Can you work these out from the model? Positions are in its coordinate system, mm. Face numbers are marked on the shaded views. Give positions to 0.01 mm unless a question says otherwise; leave off trailing zeros. Loops run counter-clockwise (first coordinate to the right, second up) from the corner with the lowest first, then second, coordinate; pieces in that order, holes last. Notation, with made-up numbers: (16, 54) - (51, 54) arc R14 ccw to (51, 75) - close; hole circle Ø4 at (14, 65). An arc over 180 degrees is marked (long way). Answer as a JSON object with one key per item and string values. Group by question number.
Item 1: Thinking about a two-plate mould opening in Y: for the marked faces 1, 2 and 3, which applies, pulls with the +Y half, pulls with the -Y half, needs draft (parallel to the pull), parting line crosses it, or undercut?
Item 2: Suppose I cut it at C-C on x = 0. Write out the boundary of the cut face in (y, z).
Item 3: Suppose I cut it at D-D on x = 22. Write out the boundary of the cut face in (y, z), and give its area (3 significant figures).
Item 4: Will these pins go through, and if not, where does the flat tip stop? pin 1 (10 mm diameter, centred on x = 18.5, y = 19, fed in from -Z); pin 2 (4 mm diameter, centred on x = 15, y = 9, fed in from -Z); pin 3 (5 mm diameter, centred on y = 12.5, z = -2, fed in from -X).
Item 5: Suppose I cut it at B-B on y = 5.5. Count the separate pieces of the cut face and the enclosed holes in it, and give its area (3 significant figures).
Item 6: Please list where these lines run through material, in increasing order: L1, parallel to Z at x = 0, y = 14.5; L2, parallel to Y at x = 10.5, z = -23; L3, parallel to X at y = 21.5, z = -18.
Item 7: Suppose I cut it at A-A on z = 0. Write out the boundary of the cut face in (x, y).
from build123d import *

# Parameters (mm, degrees)
F0_R     = 25.4
F1_DEPTH = 6.35
F3_R     = 22.225
F4_DEPTH = 19.05
F5_R     = 25.4
F6_DEPTH = 6.35
F8_D     = 3.175
F9_D     = 12.7


with BuildPart() as f1:
    # F0 (on Front) → F1 (new body)
    with BuildSketch(Plane.XZ):
        with Locations((0.658478, 0)):
            Circle(F0_R)
    extrude(amount=F1_DEPTH)

    # F3 (on face) → F4 (join)
    with BuildSketch(Plane(origin=(0, 0, 0), x_dir=(-1, 0, 0), z_dir=(0, 1, 0))):
        with Locations((-0.658478, 0)):
            Circle(F3_R)
    extrude(amount=F4_DEPTH)

    # F5 (on face) → F6 (join)
    with BuildSketch(Plane(origin=(0, 19.05, 0), x_dir=(-1, 0, 0), z_dir=(0, 1, 0))):
        with Locations((-0.658478, 0)):
            Circle(F5_R)
    extrude(amount=F6_DEPTH)

    # F8 (through all)
    with Locations(Plane.XZ.offset(6.35)):
        with Locations((0.658478, 19.05), (19.708478, 0), (0.658478, -19.05), (-18.391522, 0)):
            Hole(F8_D / 2)

    # F9 (through all)
    with Locations(Plane.XZ.offset(6.35)):
        with Locations((0.658478, 0)):
            Hole(F9_D / 2)


solid = f1.part
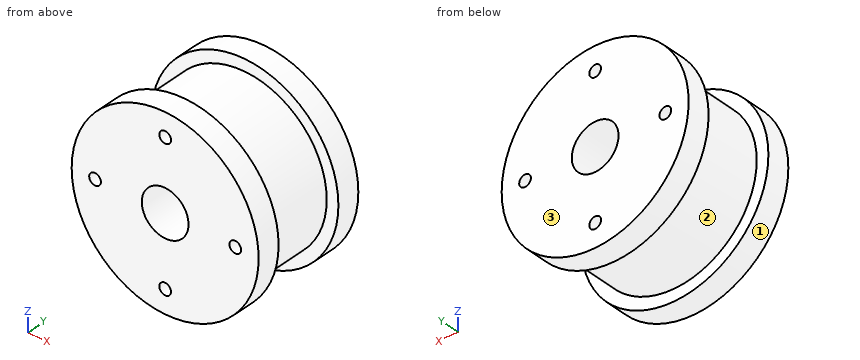
Worked out:
{
 "1": {"face 1": "needs draft", "face 2": "undercut", "face 3": "pulls with the +Y half"},
 "2": {"outline": "(-6.35, -25.39) - (0, -25.39) - (0, -22.22) - (19.05, -22.22) - (19.05, -25.39) - (25.4, -25.39) - (25.4, -20.49) - (-6.35, -20.49) - close; (-6.35, -17.61) - (25.4, -17.61) - (25.4, -6.32) - (-6.35, -6.32) - close; (-6.35, 6.32) - (25.4, 6.32) - (25.4, 17.61) - (-6.35, 17.61) - close; (-6.35, 20.49) - (25.4, 20.49) - (25.4, 25.39) - (19.05, 25.39) - (19.05, 22.22) - (0, 22.22) - (0, 25.39) - (-6.35, 25.39) - close"},
 "3": {"outline": "(-6.35, -13.77) - (0, -13.77) - (0, -6.2) - (19.05, -6.2) - (19.05, -13.77) - (25.4, -13.77) - (25.4, 13.77) - (19.05, 13.77) - (19.05, 6.2) - (0, 6.2) - (0, 13.77) - (-6.35, 13.77) - close", "area": "586 mm2"},
 "4": {"pin 1": "stops at z = -21.91", "pin 2": "stops at z = -18.48", "pin 3": "stops at x = -21.57"},
 "5": {"separate pieces": "1", "enclosed holes": "5", "area": "1,390 mm2"},
 "6": {"L1": "z = -22.22 to -20.49, -17.61 to -6.32, 6.32 to 17.61, 20.49 to 22.22", "L2": "y = -6.35 to 0, 19.05 to 25.4", "L3": "x = -17.26 to -0.53, 1.85 to 18.58"},
 "7": {"outline": "(-24.74, -6.35) - (-19.98, -6.35) - (-19.98, 25.4) - (-24.74, 25.4) - (-24.74, 19.05) - (-21.57, 19.05) - (-21.57, 0) - (-24.74, 0) - close; (-16.8, -6.35) - (-5.69, -6.35) - (-5.69, 25.4) - (-16.8, 25.4) - close; (7.01, -6.35) - (18.12, -6.35) - (18.12, 25.4) - (7.01, 25.4) - close; (21.3, -6.35) - (26.06, -6.35) - (26.06, 0) - (22.88, 0) - (22.88, 19.05) - (26.06, 19.05) - (26.06, 25.4) - (21.3, 25.4) - close"}
}
